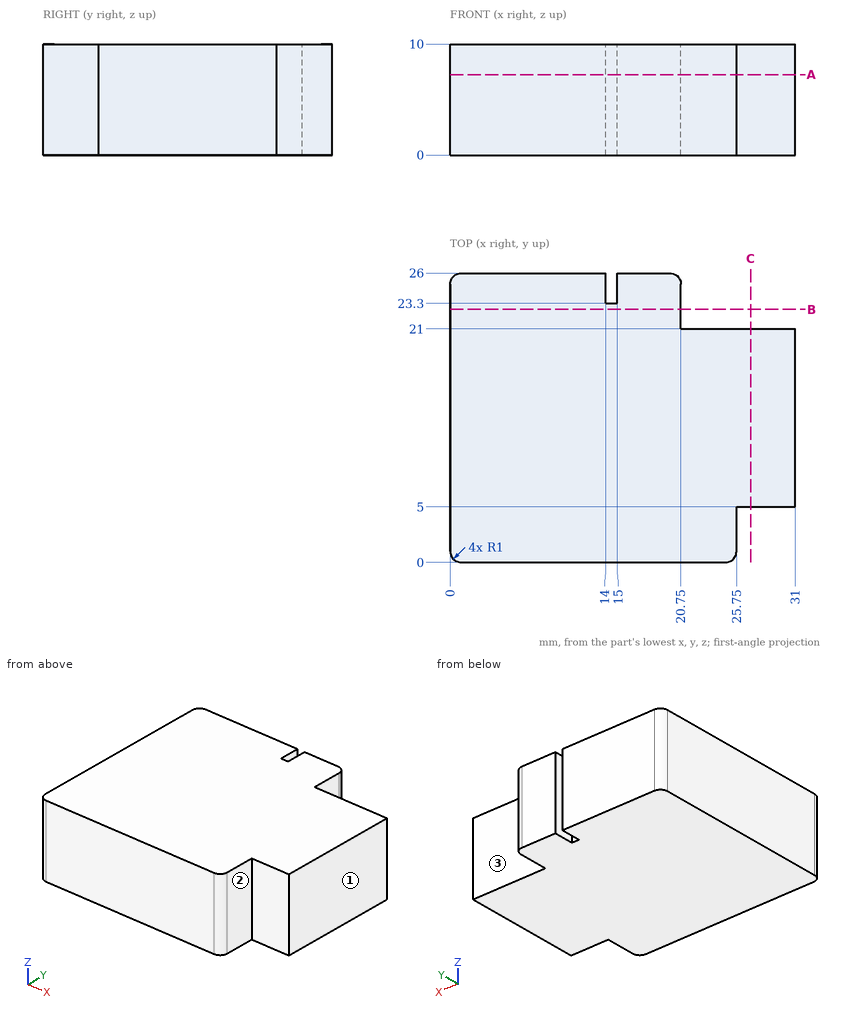
Verification items for this drawing (mm, ordinates from the low corner). A direction names the side the tool comes from. Coordinates: 2 decimals unless noted, no trailing zeros. Write each loop counter-clockwise with the first axis right and the second up, starting at its lowest first coordinate (ties: lowest second). Pieces come first, ordered by that corner, then holes. Notation, with made-up numbers: (74.5, 58.5) -> (111.5, 58.5) arc R12 ccw to (111.5, 62.5) -> close; hole circle Ø4 at (31.5, 39.25). An arc over 180 degrees is marked (long way). One line per item, written item: value. Start each with the question number.
Q1. Cross-section at A-A on z = 7.25. Enter the section's corners in (x, y).
Q2. Cross-section at B-B on y = 22.75. Enter the section's corners in (x, z), and give its area (4 significant figures).
Q3. Thickness scan on L1, parallel to X at y = 24.75, z = 5.25; L2, parallel to Y at x = 24.5, z = 2.5; L3, parallel to X at y = 3.25, z = 9.25. Record the ranges inside material, lowest first. Write a range as from..to.
Q4. Go/stop test with flat-tipped pins: P1, Ø2.5, axis at x = 27.5, z = 5, coming from the -Y side; P2, Ø2, axis at y = 24, z = 4.5, coming from the +X side; P3, Ø1, axis at y = 3, z = 8.5, coming from the +X side. Record where each tip stops, or that it passes through.
Q5. Cross-section at C-C on x = 27. Enter the section's corners in (y, z).
Q6. Access from +Z, -Z, +X, -X, +Y, -Y to the whole of each face (thin tool, end or side, straight path). Record for the marked faces 1, 2 and 3.
Checked values:
1. outline: (0, 1) arc R1 ccw to (1, 0) -> (24.75, 0) arc R1 ccw to (25.75, 1) -> (25.75, 5) -> (31, 5) -> (31, 21) -> (20.75, 21) -> (20.75, 25) arc R1 ccw to (19.75, 26) -> (15, 26) -> (15, 23.3) -> (14, 23.3) -> (14, 26) -> (1, 26) arc R1 ccw to (0, 25) -> close
2. outline: (0, 0) -> (20.75, 0) -> (20.75, 10) -> (0, 10) -> close
2. area: 207.5 mm²
3. L1: x = 0..14, 15..20.75
3. L2: y = 0..21
3. L3: x = 0..25.75
4. P1: stops at y = 5
4. P2: stops at x = 20.75
4. P3: stops at x = 25.75
5. outline: (5, 0) -> (21, 0) -> (21, 10) -> (5, 10) -> close
6. face 1: +Z, -Z, +X, +Y, -Y
6. face 2: +Z, -Z, +X, -Y
6. face 3: +Z, -Z, +X, +Y
